from build123d import *

# Parameters (mm, degrees)
SKETCH2_R           = 3.5
BOSS_EXTRUDE1_DEPTH = 31
SKETCH4_R           = 3.5
SKETCH4_W           = 4.5
SKETCH4_H           = 4.5
CUT_EXTRUDE1_DEPTH  = 10
SKETCH7_R           = 1.1
CUT_EXTRUDE2_DEPTH  = 6


with BuildPart() as part:
    # Sketch2 → Boss-Extrude1 (new body)
    with BuildSketch(Plane.XY):
        Circle(SKETCH2_R)
    extrude(amount=BOSS_EXTRUDE1_DEPTH)

    # Sketch4 → Cut-Extrude1 (cut)
    with BuildSketch(Plane(origin=(0, 0, 0), x_dir=(-1, 0, 0), z_dir=(0, 0, -1))):
        Circle(SKETCH4_R)
        Rectangle(SKETCH4_W, SKETCH4_H, mode=Mode.SUBTRACT)
    extrude(amount=-CUT_EXTRUDE1_DEPTH, mode=Mode.SUBTRACT)

    # Sketch7 → Cut-Extrude2 (cut)
    with BuildSketch(Plane.XY.offset(31)):
        Circle(SKETCH7_R)
    extrude(amount=-CUT_EXTRUDE2_DEPTH, mode=Mode.SUBTRACT)


solid = part.part
For this review, take the finished solid that the model builds, in its own axes (mm). A direction names the side the tool comes from. Round coordinates to 2 decimals unless told otherwise and drop trailing zeros. Loops run counter-clockwise (first coordinate to the right, second up) from the corner with the lowest first, then second, coordinate; pieces in that order, holes last. Notation, with made-up numbers: (26.25, 38.25) - (38.25, 38.25) arc R30 ccw to (38.25, 64.25) - close; hole circle Ø6 at (1, 77.5). An arc over 180 degrees is marked (long way). One line per item, written item: value. Start each with the question number.
Item 1: Clearance check with flat-ended pins moving along their axes: pin 1 Ø3 at (x, z) = (2.5, 16.5) entering from +Y; pin 2 Ø3.5 at (y, z) = (1, 6.5) entering from +X; pin 3 Ø1.3 at (y, z) = (0, 3.5) entering from -X. State where each tip first meets the part, or that it passes through.
Item 2: Take a section at D-D (x = -1.5). Give the boundary of the cut face in (y, z).
Item 3: Take a section at A-A (y = 0). Give the boundary of the cut face in (x, z), plus the area to 3 significant figures.
Item 4: For L1, parallel to Y at x = 0, z = 26.3; L2, parallel to Z at x = 2.5, y = -1.75; L3, parallel to Y at x = 2, z = 1.5, list the stretches that pass through material, from the lowest coordinate up.
Item 5: The part is to be moulded in two halves that separate along Y. For faces 4 (the flat face through (-2.25, 0, 5)), 5 (the cylindrical face through (1.05, 0.33, 28.04)), 6 (the flat face through (0, 0, 25)), 7 (the cylindrical face through (3.233, -1.341, 20.353)), say which applies: +Y half, -Y half, draft (parallel to the pull), parting line (faces both ways), or undercut.
Item 6: For faces 1 (the flat face through (2.25, 0, 5)), 2 (the flat face through (0, 2.25, 5)), 3 (the flat face through (0, -2.25, 5)), list the 3-axis set-ups (+Z, -Z, +X, -X, +Y, -Y) from which the entire face can be reached by the end or side of a thin tool; tool diameter is ignored.
Item 7: Take a section at C-C (z = 4.5). Give the boundary of the cut face in (x, y), plus the area to 4 significant figures.
Answer below:
1. pin 1: stops at y = 3.35
1. pin 2: stops at x = 2.25
1. pin 3: stops at x = -2.25
2. outline: (-3.16, 10) - (-2.25, 10) - (-2.25, 0) - (2.25, 0) - (2.25, 10) - (3.16, 10) - (3.16, 31) - (-3.16, 31) - close
3. outline: (-3.5, 10) - (-2.25, 10) - (-2.25, 0) - (2.25, 0) - (2.25, 10) - (3.5, 10) - (3.5, 31) - (1.1, 31) - (1.1, 25) - (-1.1, 25) - (-1.1, 31) - (-3.5, 31) - close
3. area: 179 mm2
4. L1: y = -3.5 to -1.1, 1.1 to 3.5
4. L2: z = 10 to 31
4. L3: y = -2.25 to 2.25
5. face 4: draft
5. face 5: undercut
5. face 6: undercut
5. face 7: parting line
6. face 1: -Z, +X, +Y, -Y
6. face 2: -Z, +X, -X, +Y
6. face 3: -Z, +X, -X, -Y
7. outline: (-2.25, -2.25) - (2.25, -2.25) - (2.25, 2.25) - (-2.25, 2.25) - close
7. area: 20.25 mm2
